Source: CAD feature listing. Evaluate the final solid. Frame: model axes, mm. Face numbers are marked on the shaded views. A direction names the side the tool comes from. Give positions to 0.01 mm unless a question says otherwise; leave off trailing zeros. Order: outer loops, then holes, each group sorted by start corner. A loop starts at its lowest first (then second) coordinate and runs counter-clockwise, first axis right, second up. Notation, with made-up numbers: (-22, 1.25) - (-12, 1.25) arc R25 ccw to (-12, 21.25) - close; hole circle Ø2 at (73, -9.5). An arc over 180 degrees is marked (long way). Use CSV: the item, a comma, the result in double quotes.
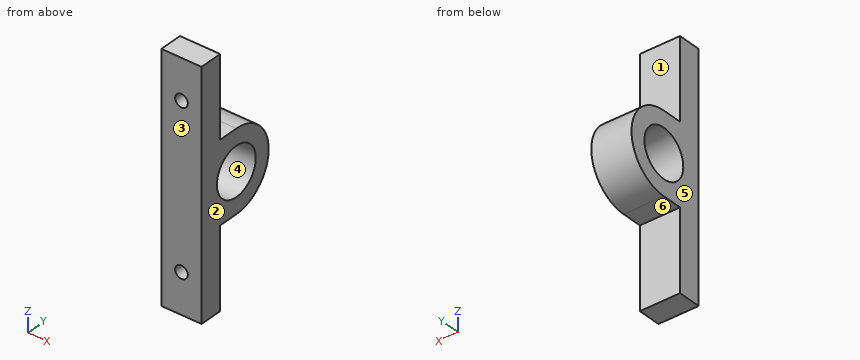
```python
from build123d import *

# Parameters (mm, degrees)
BOSS_EXTRUDE1_DEPTH = 12.7
SKETCH2_R           = 7.62500004
CUT_EXTRUDE1_DEPTH  = 82.621397317
SKETCH3_R           = 2
CUT_EXTRUDE2_DEPTH  = 7


with BuildPart() as part:
    # Sketch1 → Boss-Extrude1 (new body)
    with BuildSketch(Plane(origin=(0, 0, 0), x_dir=(0, 0, -1), z_dir=(1, 0, 0))):
        with BuildLine():
            Line((0, 0), (76.2, 0))
            Line((76.2, 0), (76.2, 7.3))
            Line((76.2, 7.3), (50.8, 7.3))
            Line((50.8, 7.3), (50.8, 13.65))
            ThreePointArc((50.8, 13.65), (38.1, 26.35), (25.4, 13.65))
            Line((25.4, 13.65), (25.4, 7.3))
            Line((25.4, 7.3), (0, 7.3))
            Line((0, 7.3), (0, 0))
        make_face()
    extrude(amount=BOSS_EXTRUDE1_DEPTH)

    # Sketch2 → Cut-Extrude1 (cut, through all)
    with BuildSketch(Plane(origin=(12.7, 0, 0), x_dir=(0, 0, -1), z_dir=(1, 0, 0))):
        with Locations((38.1, 13.65)):
            Circle(SKETCH2_R)
    extrude(amount=-CUT_EXTRUDE1_DEPTH, mode=Mode.SUBTRACT)

    # Sketch3 → Cut-Extrude2 (cut)
    with BuildSketch(Plane.XZ):
        with Locations(Location((6.35, -12.7, 0), (0, 0, 270))):
            Circle(SKETCH3_R)
        with Locations(Location((6.35, -63.5, 0), (0, 0, 270))):
            Circle(SKETCH3_R)
    extrude(amount=-CUT_EXTRUDE2_DEPTH, mode=Mode.SUBTRACT)


solid = part.part
```
Item 1: Material intervals for line 1 (Z direction, x = 4.75, y = 6.75); line 2 (X direction, y = 3.5, z = -63.5); line 3 (Y direction, x = 5.75, z = -63.5), sorted ascending. Write a range as from..to.
Filled in:
line 1,"z = -76.2..-64.7, -62.3..-41.35, -34.85..-13.9, -11.5..0"
line 2,"x = 0..4.35, 8.35..12.7"
line 3,"y = 7..7.3"
Item 2: Section B-B on x = 6.35. Return the cut outline in (y, z) (3 decimals).
Filled in:
outline,"(0, -76.2) - (7.3, -76.2) - (7.3, -50.8) - (13.65, -50.8) arc R12.7 ccw to (13.65, -25.4) - (7.3, -25.4) - (7.3, 0) - (0, 0) - (0, -10.7) - (7, -10.7) - (7, -14.7) - (0, -14.7) - (0, -61.5) - (7, -61.5) - (7, -65.5) - (0, -65.5) - close; hole circle Ø15.25 at (13.65, -38.1)"
Item 3: Section A-A on z = -38.1. Return the cut outline in (x, y) (3 decimals), then the cut area to 3 significant figures.
Filled in:
outline,"(0, 0) - (12.7, 0) - (12.7, 6.025) - (0, 6.025) - close; (0, 21.275) - (12.7, 21.275) - (12.7, 26.35) - (0, 26.35) - close"
area,"141 mm2"
Item 4: Section D-D on z = -63.5. Return the cut outline in (x, y).
Filled in:
outline,"(0, 0) - (4.35, 0) - (4.35, 7) - (8.35, 7) - (8.35, 0) - (12.7, 0) - (12.7, 7.3) - (0, 7.3) - close"
Item 5: Set-up query: the marked faces 5 and 6. Return all of +Z, -Z, +X, -X, +Y, -Y with unobstructed straight access to the full face (end or side cutting, diameter ignored); none if empty.
Filled in:
face 5,"+Z, -Z, -X, +Y, -Y"
face 6,"-Z, +X, -X, +Y"
Item 6: Section C-C on y = 16.75. Return the cut outline in (x, z).
Filled in:
outline,"(0, -50.42) - (12.7, -50.42) - (12.7, -45.07) - (0, -45.07) - close; (0, -31.13) - (12.7, -31.13) - (12.7, -25.78) - (0, -25.78) - close"
Item 7: Mould query, pull axis Y, two halves, no side actions, for the marked faces 1, 2, 3 and 4. Classes: released by +Y, released by -Y, zero draft, split by the parting line, or undercut.
Filled in:
face 1,"released by +Y"
face 2,"zero draft"
face 3,"released by -Y"
face 4,"undercut"
Item 8: First-contact query: pin 1 (6.5 mm diameter, centred on x = 8.5, z = -18, fed in from +Y); pin 2 (3 mm diameter, centred on x = 10.5, y = 14, fed in from -Z); pin 3 (10 mm diameter, centred on y = 20, z = -18, fed in from +X); pin 4 (1 mm diameter, centred on x = 9.5, y = 13, fed in from +Z). Flat tips, straight axial feed; report the tip coordinate or a pass-through.
Filled in:
pin 1,"stops at y = 7.3"
pin 2,"stops at z = -50.8"
pin 3,"passes through"
pin 4,"stops at z = -25.4"
